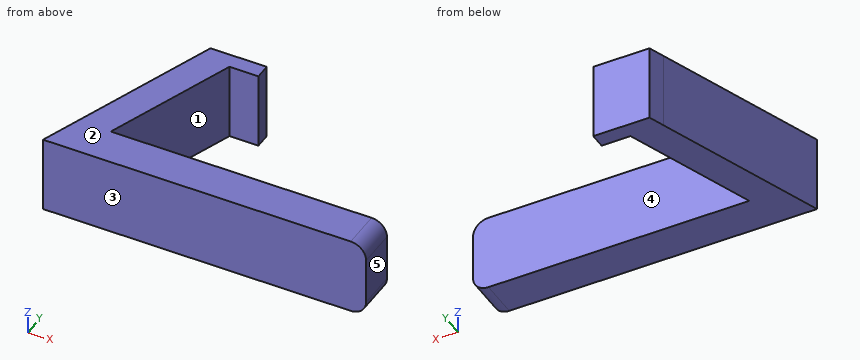
```python
from build123d import *

# Parameters (mm, degrees)
SKETCH1_W           = 50.8
SKETCH1_H           = 12.7
BOSS_EXTRUDE1_DEPTH = 6.35
FILLET1_R           = 2.54
BOSS_EXTRUDE2_DEPTH = 12.7
BOSS_EXTRUDE3_DEPTH = 12.7


with BuildPart() as part:
    # Sketch1 → Boss-Extrude1 (new body)
    with BuildSketch(Plane(origin=(0, 0, 0), x_dir=(1, 0, 0), z_dir=(0, 1, 0))):
        with Locations((25.4, 6.35)):
            Rectangle(SKETCH1_W, SKETCH1_H)
    extrude(amount=BOSS_EXTRUDE1_DEPTH)

    # Fillet1
    fillet1_edges = [part.edges().sort_by_distance(p)[0] for p in [
        (50.8, 3.175, -12.7),
        (50.8, 3.175, 0),
    ]]
    fillet(fillet1_edges, radius=FILLET1_R)

    # Sketch3 → Boss-Extrude2 (add)
    with BuildSketch(Plane.XY):
        Polygon((-2.311210988, 0), (7.858117358, 27.94), (13.264140442, 27.94), (3.094812097, 0), align=None)
    extrude(amount=-BOSS_EXTRUDE2_DEPTH)

    # Sketch4 → Boss-Extrude3 (add)
    with BuildSketch(Plane.XY):
        Polygon((7.858117358, 27.94), (18.018117358, 27.94), (18.018117358, 30.48), (8.782601753, 30.48), align=None)
    extrude(amount=-BOSS_EXTRUDE3_DEPTH)


solid = part.part
```
For this review, take the finished solid that the model builds, in its own axes (mm). Face numbers are marked on the shaded views. A direction names the side the tool comes from. Coordinates: 2 decimals unless noted, no trailing zeros. Loops run counter-clockwise (first coordinate to the right, second up) from the corner with the lowest first, then second, coordinate; pieces in that order, holes last. Notation, with made-up numbers: (66, -19) -> (79, -19) arc R31 cw to (79, 9) -> close; hole circle Ø1 at (-21.5, -6.5). An arc over 180 degrees is marked (long way). Return JSON: item names as keys, results as strings. Group by question number.
(1) For pin 1 Ø0.8 at (y, z) = (29.5, -5.5) entering from +X; pin 2 Ø6 at (y, z) = (23, -10.5) entering from +X; pin 3 Ø6 at (x, z) = (35, -2.5) entering from +Y, all flat-tipped, find the tip position at first contact; note any pin that passes through.
(2) To check wall thickness, follow L1, parallel to Y at x = 28.5, z = -0.75; L2, parallel to Y at x = 14.5, z = -0.75. State the ranges of each line that lie inside material, in increasing order.
(3) Consider section D-D, the plane z = -11.25. Give the boundary of the cut face in (x, y), plus the area to 3 significant figures.
(4) Tool access review of the marked faces 1 and 2: name each direction out of +Z, -Z, +X, -X, +Y, -Y from which nothing blocks a thin tool from reaching the whole face with its end or side.
(5) Consider section A-A, the plane z = -8.25. Give the boundary of the cut face in (x, y).
(6) Consider section B-B, the plane y = 3.5. Give the boundary of the cut face in (x, z).
(7) Mouldability with a two-part tool opening along Y and no side actions: class the marked faces 3, 4 and 5 as pulls with the +Y half, pulls with the -Y half, needs draft (parallel to the pull), parting line crosses it, or undercut.
(8) Consider section C-C, the plane x = 32.5. Give the boundary of the cut face in (y, z).
Results below:
{
 "1": {"pin 1": "stops at x = 18.02", "pin 2": "stops at x = 12.56", "pin 3": "stops at y = 6.35"},
 "2": {"L1": "y = 0 to 6.35", "L2": "y = 0 to 6.35, 27.94 to 30.48"},
 "3": {"outline": "(-2.31, 0) -> (50.55, 0) -> (50.55, 6.35) -> (5.41, 6.35) -> (13.26, 27.94) -> (18.02, 27.94) -> (18.02, 30.48) -> (8.78, 30.48) -> close", "area": "470 mm2"},
 "4": {"face 1": "+Z, -Z, +X", "face 2": "+Z, +X, -X, +Y, -Y"},
 "5": {"outline": "(-2.31, 0) -> (50.8, 0) -> (50.8, 6.35) -> (5.41, 6.35) -> (13.26, 27.94) -> (18.02, 27.94) -> (18.02, 30.48) -> (8.78, 30.48) -> close"},
 "6": {"outline": "(-1.04, -12.7) -> (48.26, -12.7) arc R2.54 ccw to (50.8, -10.16) -> (50.8, -2.54) arc R2.54 ccw to (48.26, 0) -> (-1.04, 0) -> close"},
 "7": {"face 3": "pulls with the -Y half", "face 4": "undercut", "face 5": "needs draft"},
 "8": {"outline": "(0, -12.7) -> (6.35, -12.7) -> (6.35, 0) -> (0, 0) -> close"}
}
